Study the drawing (mm; zero at the part's minimum x, y, z) and answer. Give positions to 0.01 mm unless a question says otherwise; leave off trailing zeros. Order: outer loops, then holes, each group sorted by start corner. A loop starts at its lowest first (then second) coordinate and runs counter-clockwise, first axis right, second up. Notation, with made-up numbers: (11, 14.5) - (51, 14.5) arc R20 cw to (51, 36.5) - close; hole circle Ø7 at (-30.75, 48). An arc over 180 degrees is marked (long way). Use CSV: the item, a comma, the result in double quotes.
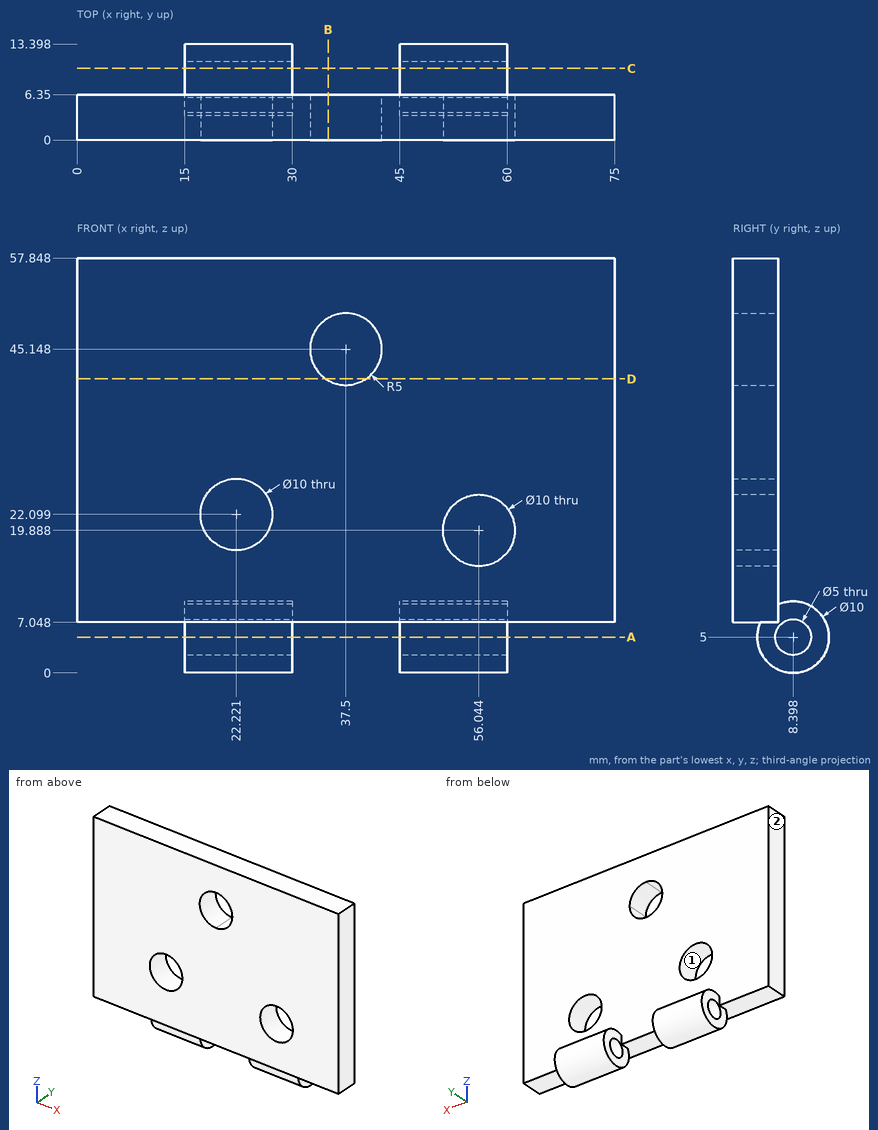
Item 1: Find the intervals of material crossed by line 1 along Y through (x, z) = (22, 5); line 2 along Z through (x, y) = (10.5, 4.25); line 3 along Y through (x, z) = (20, 37.5), in increasing order.
Taken from the geometry:
line 1,"3.4 to 5.9, 10.9 to 13.4"
line 2,"7.05 to 57.85"
line 3,"0 to 6.35"
Item 2: The part is cut by section A-A (z = 5). Give the vertices of the cut face in (x, y).
Taken from the geometry:
outline,"(15, 3.4) - (30, 3.4) - (30, 5.9) - (15, 5.9) - close; (15, 10.9) - (30, 10.9) - (30, 13.4) - (15, 13.4) - close; (45, 3.4) - (60, 3.4) - (60, 5.9) - (45, 5.9) - close; (45, 10.9) - (60, 10.9) - (60, 13.4) - (45, 13.4) - close"
Item 3: The part is cut by section C-C (y = 10). Give the vertices of the cut face in (x, z).
Taken from the geometry:
outline,"(15, 0.26) - (30, 0.26) - (30, 3.08) - (15, 3.08) - close; (15, 6.92) - (30, 6.92) - (30, 9.74) - (15, 9.74) - close; (45, 0.26) - (60, 0.26) - (60, 3.08) - (45, 3.08) - close; (45, 6.92) - (60, 6.92) - (60, 9.74) - (45, 9.74) - close"
Item 4: Each of these flat-tipped pins is pushed along its axis until it touches: pin 1 (3 mm diameter, centred on x = 66, z = 16.5, fed in from +Y); pin 2 (4 mm diameter, centred on x = 58, y = 2.5, fed in from -Z); pin 3 (5 mm diameter, centred on x = 23, y = 11.5, fed in from -Z); pin 4 (9 mm diameter, centred on x = 56.04, z = 19.89, fed in from -Y). Where does it stop, or does it pass through?
Taken from the geometry:
pin 1,"y = 6.35"
pin 2,"z = 1.87"
pin 3,"z = 0.04"
pin 4,"through"
Item 5: The part is cut by section B-B (x = 35). Give the vertices of the cut face in (y, z).
Taken from the geometry:
outline,"(0, 7.05) - (6.35, 7.05) - (6.35, 40.82) - (0, 40.82) - close; (0, 49.48) - (6.35, 49.48) - (6.35, 57.85) - (0, 57.85) - close"
Item 6: The part is cut by section D-D (z = 41). Give the vertices of the cut face in (x, y), and give its area (3 significant figures).
Taken from the geometry:
outline,"(0, 0) - (34.71, 0) - (34.71, 6.35) - (0, 6.35) - close; (40.29, 0) - (75, 0) - (75, 6.35) - (40.29, 6.35) - close"
area,"441 mm^2"
Item 7: The mould has two halves that part along Z. Classify the marked faces 1 and 2: +Z half, -Z half, draft (parallel to the pull), parting line (faces both ways), or undercut.
Taken from the geometry:
face 1,"undercut"
face 2,"draft"
